Model file for the job. Use its own axes, mm. A direction names the side the tool comes from. Give positions to 0.01 mm unless a question says otherwise; leave off trailing zeros. Loops run counter-clockwise (first coordinate to the right, second up) from the corner with the lowest first, then second, coordinate; pieces in that order, holes last. Notation, with made-up numbers: M 80,5.5 L 136,5.5 A24 ccw 136,16.5 Z; hole C 29.5,25.5 d10. An arc over 180 degrees is marked long. Answer in a Markdown table with one row per item.
```python
from build123d import *

# Parameters (mm, degrees)
SKETCH1_R           = 1.500000001
SKETCH1_R_2         = 1.5
BOSS_EXTRUDE1_DEPTH = 12
SKETCH6_W           = 31
SKETCH6_H           = 1
BOSS_EXTRUDE2_DEPTH = 1
SKETCH7_W           = 31
SKETCH7_H           = 1
BOSS_EXTRUDE3_DEPTH = 1
SKETCH8_W           = 28
SKETCH8_H           = 1
BOSS_EXTRUDE4_DEPTH = 0.75
SKETCH9_W           = 28
SKETCH9_H           = 1
BOSS_EXTRUDE5_DEPTH = 0.75
CUT_EXTRUDE5_DEPTH  = 41
BOSS_EXTRUDE6_DEPTH = 5


with BuildPart() as part:
    # Sketch1 → Boss-Extrude1 (new body)
    with BuildSketch(Plane(origin=(0, 0, 0), x_dir=(1, 0, 0), z_dir=(0, 1, 0))):
        with BuildLine():
            Line((-206.901303799, 210.544296342), (-178.864917553, 182.014262429))
            ThreePointArc((-178.864917553, 182.014262429), (-211.248528729, 143.160707083), (-235.332727793, 98.683202756))
            ThreePointArc((-235.332727793, 98.683202756), (-249.691560201, 52.678328759), (-255.14463702, 4.794213931))
            Line((-255.14463702, 4.794213931), (-255.14463702, 2.779626552))
            Line((-255.14463702, 2.779626552), (-259.725038425, 2.779626552))
            Line((-259.725038425, 2.779626552), (-259.725038425, 4.938563385))
            Line((-259.725038425, 4.938563385), (-258.586614607, 25.913112119))
            Line((-258.586614607, 25.913112119), (-289.472992235, 26.886483517))
            Line((-289.472992235, 26.886483517), (-290.232709847, 5.900000013))
            Line((-290.232709847, 5.900000013), (-290.232709847, 2.779626551))
            Line((-290.232709847, 2.779626551), (-295.127762341, 2.779626551))
            Line((-295.127762341, 2.779626551), (-295.127762341, 6.054265565))
            ThreePointArc((-295.127762341, 6.054265565), (-271.03936796, 116.93892103), (-206.901303799, 210.544296342))
        make_face()
        with Locations(Location((-205.923171716, 204.555428223, 0), (0, 0, 270))):
            Circle(SKETCH1_R, mode=Mode.SUBTRACT)
        with Locations(Location((-182.123524849, 182.048793456, 0), (0, 0, 270))):
            Circle(SKETCH1_R_2, mode=Mode.SUBTRACT)
        with Locations(Location((-289.472992235, 30.413510705, 0), (0, 0, 270))):
            Circle(SKETCH1_R_2, mode=Mode.SUBTRACT)
        with Locations(Location((-256.189573648, 27.390600482, 0), (0, 0, 270))):
            Circle(SKETCH1_R_2, mode=Mode.SUBTRACT)
        with Locations(Location((-237.445118633, 99.492127605, 0), (0, 0, 270))):
            Circle(SKETCH1_R_2, mode=Mode.SUBTRACT)
        with Locations(Location((-268.833815416, 112.841343478, 0), (0, 0, 270))):
            Circle(SKETCH1_R_2, mode=Mode.SUBTRACT)
        Polygon((-288.286547304, 34.069084362), (-258.033222279, 30.008925637), (-254.767009525, 50.758854735), (-285.491553173, 54.882253531), align=None, mode=Mode.SUBTRACT)
        Polygon((-283.612878523, 61.915838046), (-253.89939669, 54.933619681), (-248.631031599, 75.267631401), (-278.809043274, 82.359007245), align=None, mode=Mode.SUBTRACT)
        Polygon((-276.255921554, 89.176800074), (-247.361344598, 79.340855863), (-240.142390382, 99.066838813), (-269.488694715, 109.056554622), align=None, mode=Mode.SUBTRACT)
        Polygon((-229.967759139, 120.819849226), (-238.977493449, 101.844802692), (-266.671759318, 115.77418308), (-257.235727442, 134.534814797), align=None, mode=Mode.SUBTRACT)
        Polygon((-217.141868251, 142.590375773), (-227.952465343, 124.580414811), (-254.16244031, 141.134484167), (-242.948393328, 158.889628499), align=None, mode=Mode.SUBTRACT)
        Polygon((-202.261755682, 163.008777697), (-214.772333152, 146.135332444), (-239.248466479, 165.159498585), (-226.362501502, 181.741172494), align=None, mode=Mode.SUBTRACT)
        Polygon((-185.566118156, 181.787515485), (-199.72829266, 166.274278663), (-222.071098467, 187.621756348), (-207.634972794, 202.873245989), align=None, mode=Mode.SUBTRACT)
    extrude(amount=BOSS_EXTRUDE1_DEPTH)

    # Sketch6 → Boss-Extrude2 (add)
    with BuildSketch(Plane(origin=(2.241673695, 0, -2.346191939), x_dir=(0.7230281012906209, 0, 0.6908186192801116), z_dir=(-0.6908186192801116, 0, 0.7230281012906209))):
        with Locations((-275.013127173, 11.5)):
            Rectangle(SKETCH6_W, SKETCH6_H)
    extrude(amount=BOSS_EXTRUDE2_DEPTH)

    # Sketch7 → Boss-Extrude3 (add)
    with BuildSketch(Plane(origin=(-12.265517311, 0, 12.83739819), x_dir=(-0.7230281012906384, 0, -0.6908186192800932), z_dir=(0.6908186192800932, 0, -0.7230281012906384))):
        with Locations((274.725391583, 11.5)):
            Rectangle(SKETCH7_W, SKETCH7_H)
    extrude(amount=BOSS_EXTRUDE3_DEPTH)

    # Sketch8 → Boss-Extrude4 (add)
    with BuildSketch(Plane(origin=(-12.265517311, 0, 12.83739819), x_dir=(-0.7230281012906384, 0, -0.6908186192800932), z_dir=(0.6908186192800932, 0, -0.7230281012906384))):
        with Locations((274.725391583, 0.5)):
            Rectangle(SKETCH8_W, SKETCH8_H)
    extrude(amount=BOSS_EXTRUDE4_DEPTH)

    # Sketch9 → Boss-Extrude5 (add)
    with BuildSketch(Plane(origin=(2.241673695, 0, -2.346191939), x_dir=(0.7230281012906209, 0, 0.6908186192801116), z_dir=(-0.6908186192801116, 0, 0.7230281012906209))):
        with Locations((-274.86046651, 0.5)):
            Rectangle(SKETCH9_W, SKETCH9_H)
    extrude(amount=BOSS_EXTRUDE5_DEPTH)

    # Sketch10 → Cut-Extrude5 (cut)
    with BuildSketch(Plane.ZY.offset(295.127762341)):
        Polygon((-2.779626551, 12), (-2.779626551, 8), (-12.781334045, 9.40564832), (-12.781334045, 2.59435168), (-2.779626551, 4), (-2.779626551, 0), (4.575602147, 0), (4.575602147, 12), align=None)
    extrude(amount=-CUT_EXTRUDE5_DEPTH, mode=Mode.SUBTRACT)

    # Sketch12 → Boss-Extrude6 (add)
    with BuildSketch(Plane(origin=(-206.901303799, 0, -210.544296342), x_dir=(-0.7132504491210117, 0, 0.700909264333605), z_dir=(-0.700909264333605, 0, -0.7132504491210117))):
        Polygon((0, 12), (0, 8), (-10, 9.417744688), (-10, 2.617744688), (0, 4.035489376), (0, 0), (0.901744135, 0), (0.901744135, 12), align=None)
    boss_extrude6 = extrude(amount=-BOSS_EXTRUDE6_DEPTH)

    # Mirror2: Boss-Extrude6 across plane
    add(boss_extrude6.mirror(Plane(origin=(-192.883118513, 0, -196.27928736), x_dir=(-0.7132504491210118, 0, 0.7009092643336048), z_dir=(-0.700909264333605, 0, -0.7132504491210117))))


solid = part.part
```
(1) Saw through at C-C, the plane x = -262.5. Give the cut face in (y, z).
Established:
| item | result |
|---|---|
| outline | M 0,-135.02 L 12,-135.02 L 12,-124.07 L 0,-124.07 Z; M 0,-113.68 L 12,-113.68 L 12,-106.68 L 0,-106.68 Z; M 0,-84.49 L 12,-84.49 L 12,-78.53 L 0,-78.53 Z; M 0,-56.95 L 12,-56.95 L 12,-51.8 L 0,-51.8 Z; M 0,-30.61 L 12,-30.61 L 12,-26.04 L 0,-26.04 Z |
(2) Wall check: L1, parallel to Z at x = -208.5, y = 4; L2, parallel to X at y = 3, z = -128.5; L3, parallel to Z at x = -237, y = 2.25. Give the ranges that are in metal, low to high.
Established:
| item | result |
|---|---|
| L1 | z = -208.96 to -201.96, -174.66 to -167.86, -154.6 to -147.14 |
| L2 | x = -265.75 to -260.27, -245.24 to -234.16, -225.6 to -220.47 |
| L3 | z = -175.98 to -168.05, -163.41 to -155.13, -130.29 to -124.36, -106.01 to -100.92, -98.06 to -94.61 |
(3) Which spindle directions (+Z, -Z, +X, -X, +Y, -Y) get a long thin tool onto all of the face, cutting with end or side? Do faces 1 (the flat face through (-201.557, 3.317, -212.34)), 2 (the flat face through (-210.5, 1, -177.1)), 3 (the flat face through (-272.825, 5.916, -99.256)), 4 (the flat face through (-289.763, 5.916, -18.872)), 5 (the flat face through (-201.66, 8.7, -212.24)). Say none if no direction does.
Established:
| item | result |
|---|---|
| face 1 | -Y |
| face 2 | none |
| face 3 | +Y, -Y |
| face 4 | +Z, +Y, -Y |
| face 5 | +Y |
(4) Saw through at D-D, the plane x = -211.5. Give the cut face in (y, z).
Established:
| item | result |
|---|---|
| outline | M 0,-205.92 L 12,-205.92 L 12,-198.79 L 0,-198.79 Z; M 0,-178.56 L 1,-178.56 L 1,-177.52 L 11,-177.52 L 11,-178.9 L 12,-178.9 L 12,-170.19 L 0,-170.19 Z; M 0,-150.55 L 12,-150.55 L 12,-142.79 L 0,-142.79 Z |
(5) Saw through at A-A, the plane z = -38. Give the cut face in (x, y).
Established:
| item | result |
|---|---|
| outline | M -292.73,0 L -287.76,0 L -287.76,12 L -292.73,12 Z; M -256.78,0 L -252.34,0 L -252.34,12 L -256.78,12 Z |
(6) Saw through at B-B, the plane z = -132.5. Give the cut face in (x, y), and give its area (3 significant figures).
Established:
| item | result |
|---|---|
| outline | M -263.78,0 L -258.26,0 L -258.26,12 L -263.78,12 Z; M -253.19,0 L -240.49,0 L -240.49,12 L -253.19,12 Z; M -223.2,0 L -218.09,0 L -218.09,12 L -223.2,12 Z |
| area | 280 mm2 |
(7) Flat gauge pins, fed straight in: P1, Ø2, axis at y = 1, z = -3.5, coming from the +X side; P2, Ø3, axis at y = 9.5, z = -147.5, coming from the +X side; P3, Ø1.8, axis at x = -256.19, z = -27.39, coming from the +Y side; P4, Ø2, axis at y = 7.5, z = -47.5, coming from the +X side. Where does each tip first touch, or does it go through?
Established:
| item | result |
|---|---|
| P1 | stops at x = -255.14 |
| P2 | stops at x = -207.17 |
| P3 | passes through |
| P4 | stops at x = -250.54 |
(8) Mould opens along Z. For faces 6 (the flat face through (-269.91, 5.92, -52.79)), 7 (the flat face through (-257, 2, -2.78)), 8 (the flat face through (-178.753, 6.065, -189.134)) say: pulls with the +Z half, pulls with the -Z half, needs draft (parallel to the pull), parting line crosses it, or undercut.
Established:
| item | result |
|---|---|
| face 6 | undercut |
| face 7 | pulls with the +Z half |
| face 8 | pulls with the -Z half |
